```python
from build123d import *

# Parameters (mm, degrees)
SKETCH1_W                                    = 172.2
SKETCH1_H                                    = 172.2
SKETCH1_W_2                                  = 162.2
SKETCH1_H_2                                  = 162.2
BASE_DEPTH                                   = 10
LEDGES_SIZE                                  = 15
POST_DEPTH                                   = 48
MIRRORED_POSTS_AT_THE_SECOND_PLANE_C_2_DEPTH = 48
SIDE_ARM_DEPTH                               = 30
TOP_BOTTOM_ARMS_DEPTH                        = 30
SKETCH9_W                                    = 22.5
SKETCH9_H                                    = 69
BOTTOM_ARM_CUTOUT_DEPTH                      = 177.122471593


with BuildPart() as part:
    # Sketch1 → base (new body)
    with BuildSketch(Plane(origin=(0, 0, 0), x_dir=(1, 0, 0), z_dir=(0, 1, 0))):
        with Locations((0, 37)):
            Rectangle(SKETCH1_W, SKETCH1_H)
        with Locations((0, 37)):
            Rectangle(SKETCH1_W_2, SKETCH1_H_2, mode=Mode.SUBTRACT)
    extrude(amount=-BASE_DEPTH)

    # ledges
    ledges_edges = [part.edges().sort_by_distance(p)[0] for p in [
        (-81.1, -5, 44.1),
        (-81.1, -5, -118.1),
        (81.1, -5, -118.1),
        (81.1, -5, 44.1),
    ]]
    chamfer(ledges_edges, length=LEDGES_SIZE)

    # Sketch2 → post (add)
    with BuildSketch(Plane(origin=(0, 0, 0), x_dir=(1, 0, 0), z_dir=(0, 1, 0))):
        Polygon((-81.1, 103.1), (-86.1, 103.1), (-86.1, 123.1), (-66.1, 123.1), (-66.1, 118.1), (-81.1, 118.1), align=None)
    post = extrude(amount=POST_DEPTH)

    # mirrored-posts: post across plane
    add(post.mirror(Plane.XY.offset(-37)))

    # mirrored-posts at the second plane: post across plane
    add(post.mirror(Plane(origin=(0, 0, 0), x_dir=(0, 0, 1), z_dir=(1, 0, 0))))

    # mirrored-posts at the second plane copy → mirrored-posts at the second plane c 2 (add)
    with BuildSketch(Plane(origin=(0, 0, -74), x_dir=(-1, 0, 0), z_dir=(0, 1, 0))):
        Polygon((-81.1, 103.1), (-86.1, 103.1), (-86.1, 123.1), (-66.1, 123.1), (-66.1, 118.1), (-81.1, 118.1), align=None)
    extrude(amount=MIRRORED_POSTS_AT_THE_SECOND_PLANE_C_2_DEPTH)

    # Sketch7 → side-arm (add, symmetric)
    with BuildSketch(Plane.XY):
        Polygon((86.1, -7.778619134), (102.75, 12.064078182), (102.75, 32.064078182), (97.75, 32.064078182), (97.75, 13.883929354), (86.1, 0), align=None)
    side_arm = extrude(amount=SIDE_ARM_DEPTH, both=True)

    # side-arm-mirrored: side-arm across plane
    add(side_arm.mirror(Plane(origin=(0, 0, 0), x_dir=(0, 0, 1), z_dir=(1, 0, 0))))

    # Sketch8 → top-bottom-arms (add, symmetric)
    with BuildSketch(Plane(origin=(0, 0, 0), x_dir=(0, 0, -1), z_dir=(1, 0, 0))):
        Polygon((123.1, -7.778619134), (134.75, 6.105310219), (134.75, 26.105310219), (129.75, 26.105310219), (129.75, 7.925161391), (123.1, 0), align=None)
        Polygon((-49.1, -10), (-123.1, -10), (-123.1, -7.778619134), (-134.75, 6.105310219), (-134.75, 26.105310219), (-129.75, 26.105310219), (-129.75, 7.925161391), (-123.1, 0), (-49.1, 0), align=None)
    extrude(amount=TOP_BOTTOM_ARMS_DEPTH, both=True)

    # Sketch9 → bottom-arm-cutout (cut, through all)
    with BuildSketch(Plane(origin=(0, 0, 0), x_dir=(1, 0, 0), z_dir=(0, 1, 0))):
        with Locations((-18.75, -83.6)):
            Rectangle(SKETCH9_W, SKETCH9_H)
        with Locations((18.75, -83.6)):
            Rectangle(SKETCH9_W, SKETCH9_H)
    extrude(amount=-BOTTOM_ARM_CUTOUT_DEPTH, mode=Mode.SUBTRACT)


solid = part.part
```
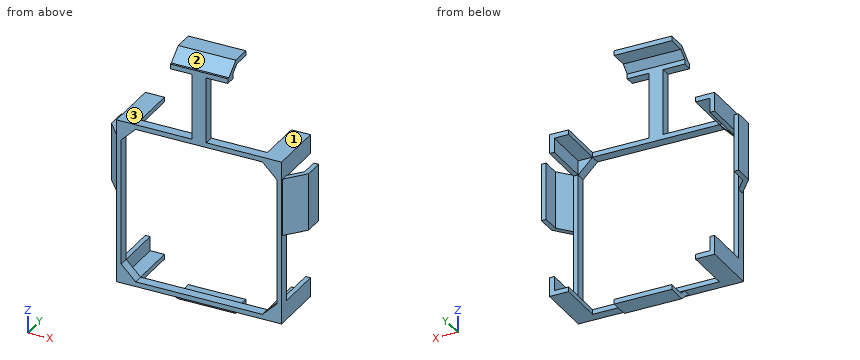
Work out the finished part from the listing and answer in its coordinate system (mm). Face numbers are marked on the shaded views. A direction names the side the tool comes from. Round coordinates to 2 decimals unless told otherwise and drop trailing zeros. Write each loop counter-clockwise with the first axis right and the second up, starting at its lowest first coordinate (ties: lowest second). Pieces come first, ordered by that corner, then holes. Notation, with made-up numbers: (20, -19) -> (33, -19) arc R24 ccw to (33, 1) -> close; hole circle Ø7 at (87.5, 30.5). An arc over 180 degrees is marked (long way). Write each question's results on one line, items separated by ' | '.
1) The part is cut by section D-D (x = -10.5). Write down the section's boundary in (y, z), and give its area (3 significant figures).
Findings:
outline: (-10, -123.1) -> (-7.78, -123.1) -> (6.11, -134.75) -> (26.11, -134.75) -> (26.11, -129.75) -> (7.93, -129.75) -> (0, -123.1) -> (0, -118.1) -> (-10, -118.1) -> close; (-10, 44.1) -> (0, 44.1) -> (0, 49.1) -> (-10, 49.1) -> close; (-10, 118.1) -> (0, 118.1) -> (0, 123.1) -> (7.93, 129.75) -> (26.11, 129.75) -> (26.11, 134.75) -> (6.11, 134.75) -> (-7.78, 123.1) -> (-10, 123.1) -> close | area: 483 mm²
2) The part is cut by section C-C (z = 0.5). Write down the section's boundary in (x, y).
Findings:
outline: (-102.75, 12.06) -> (-86.1, -7.78) -> (-86.1, -10) -> (-81.1, -10) -> (-81.1, 0) -> (-86.1, 0) -> (-97.75, 13.88) -> (-97.75, 32.06) -> (-102.75, 32.06) -> close; (81.1, -10) -> (86.1, -10) -> (86.1, -7.78) -> (102.75, 12.06) -> (102.75, 32.06) -> (97.75, 32.06) -> (97.75, 13.88) -> (86.1, 0) -> (81.1, 0) -> close
3) The part is cut by section A-A (x = -77.5). Write down the section's boundary in (y, z).
Findings:
outline: (-10, -123.1) -> (48, -123.1) -> (48, -118.1) -> (0, -118.1) -> (0, -106.7) -> (-10, -106.7) -> close; (-10, 32.7) -> (0, 32.7) -> (0, 44.1) -> (48, 44.1) -> (48, 49.1) -> (-10, 49.1) -> close
4) Which of the six approach directions +Z, -Z, +X, -X, +Y, -Y give full straight-line access (tool end or side, diameter ignored) to the marked faces 1, 2 and 3?
Findings:
face 1: +X, +Y, -Y | face 2: +Z, +X, -X, -Y | face 3: -X, +Y, -Y
5) The part is cut by section B-B (y = 35.5). Write down the section's boundary in (x, z), and give its area (3 significant figures).
Findings:
outline: (-86.1, -123.1) -> (-66.1, -123.1) -> (-66.1, -118.1) -> (-81.1, -118.1) -> (-81.1, -103.1) -> (-86.1, -103.1) -> close; (-86.1, 29.1) -> (-81.1, 29.1) -> (-81.1, 44.1) -> (-66.1, 44.1) -> (-66.1, 49.1) -> (-86.1, 49.1) -> close; (66.1, -123.1) -> (86.1, -123.1) -> (86.1, -103.1) -> (81.1, -103.1) -> (81.1, -118.1) -> (66.1, -118.1) -> close; (66.1, 44.1) -> (81.1, 44.1) -> (81.1, 29.1) -> (86.1, 29.1) -> (86.1, 49.1) -> (66.1, 49.1) -> close | area: 700 mm²
6) Flat-ended cylindrical pins translate along their axes: pin 1 (5 mm diameter, centred on y = -4.5, z = 100, fed in from -X); pin 2 (5.5 mm diameter, centred on x = 82.5, y = 30, fed in from +Z); pin 3 (4 mm diameter, centred on x = 85, y = 32, fed in from -Z); pin 4 (16.5 mm diameter, centred on x = 74.5, z = 35.5, fed in from +Y). Find the tip coordinate at first contact, or state that the pin passes through.
Findings:
pin 1: stops at x = -7.5 | pin 2: stops at z = 49.1 | pin 3: stops at z = -123.1 | pin 4: stops at y = 48
7) Consider line 1 along X through (y, z) = (39.5, 32); line 2 along Z through (x, y) = (67, 22); line 3 along Z through (x, y) = (-15, 19). Determine where each line is inside the solid, lowest interval first. Write a range as [from, to].
Findings:
line 1: x = [-86.1, -81.1], [81.1, 86.1] | line 2: z = [-123.1, -118.1], [44.1, 49.1] | line 3: z = [-134.75, -129.75], [129.75, 134.75]
